CAD build for the part. Positions are in the model's coordinates, mm. A direction names the side the tool comes from. Give positions to 0.01 mm unless a question says otherwise; leave off trailing zeros. Loops run counter-clockwise (first coordinate to the right, second up) from the corner with the lowest first, then second, coordinate; pieces in that order, holes last. Notation, with made-up numbers: M -37,-15 L -8,-15 A18 cw -8,-6 Z; hole C 10,80 d9. An arc over 180 degrees is marked long. Answer as CSV lines item,"result".
from build123d import *

# Parameters (mm, degrees)
SKETCH1_W           = 12
SKETCH1_H           = 10
BOSS_EXTRUDE1_DEPTH = 40.48
SKETCH2_OUTSIDE_W   = 22.678
SKETCH2_OUTSIDE_H   = 20.678
CUT_EXTRUDE1_DEPTH  = 10
FILLET1_R           = 1


with BuildPart() as part:
    # Sketch1 → Boss-Extrude1 (new body)
    with BuildSketch(Plane.XY):
        Rectangle(SKETCH1_W, SKETCH1_H)
    extrude(amount=-BOSS_EXTRUDE1_DEPTH)

    # Sketch2 outside → Cut-Extrude1 (cut)
    with BuildSketch(Plane.XY):
        Rectangle(SKETCH2_OUTSIDE_W, SKETCH2_OUTSIDE_H)
        with BuildLine():
            Line((-1.118033989, 1), (1.118033989, 1))
            ThreePointArc((1.118033989, 1), (0, -1.5), (-1.118033989, 1))
        make_face(mode=Mode.SUBTRACT)
    extrude(amount=-CUT_EXTRUDE1_DEPTH, mode=Mode.SUBTRACT)

    # Fillet1
    fillet1_edges = [part.edges().sort_by_distance(p)[0] for p in [
        (-6, 5, -25.24),
        (6, 5, -25.24),
    ]]
    fillet(fillet1_edges, radius=FILLET1_R)


solid = part.part
1) Band-saw the part on D-D on y = 2.5. Give the cut face in (x, z).
Answer below:
outline,"M -6,-40.48 L 6,-40.48 L 6,-10 L -6,-10 Z"
2) Flat gauge pins, fed straight in: pin 1 (2.5 mm diameter, centred on x = 0, z = -3, fed in from +Y); pin 2 (2 mm diameter, centred on x = -4, y = 2, fed in from +Z). Where does each tip first touch, or does it go through?
Answer below:
pin 1,"stops at y = 1"
pin 2,"stops at z = -10"
3) Which spindle directions (+Z, -Z, +X, -X, +Y, -Y) get a long thin tool onto all of the face, cutting with end or side? Do faces 1 (the face through (6, -1, -25)), 2 (the face through (0, 1, -5)), 3 (the face through (0, -1.5, -4.9)). Say none if no direction does.
Answer below:
face 1,"+Z, -Z, +X, +Y, -Y"
face 2,"+Z, +X, -X, +Y"
face 3,"+Z"
4) Drill centre lines: line 1 (Z direction, x = -5.5, y = -1); line 2 (X direction, y = -1, z = -9). Where is each one in solid material? Low to high. Write a range as from..to.
Answer below:
line 1,"z = -40.48..-10"
line 2,"x = -1.12..1.12"
5) Band-saw the part on A-A on x = 0. Give the cut face in (y, z), and give its area (3 significant figures).
Answer below:
outline,"M -5,-40.48 L 5,-40.48 L 5,-10 L 1,-10 L 1,0 L -1.5,0 L -1.5,-10 L -5,-10 Z"
area,"330 mm^2"
6) Band-saw the part on C-C on z = -4. Give the cut face in (x, y), and give its area (3 significant figures).
Answer below:
outline,"M -1.12,1 A1.5 ccw long 1.12,1 Z"
area,"6.29 mm^2"
7) Band-saw the part on B-B on y = 0. Give the cut face in (x, z), and give its area (3 significant figures).
Answer below:
outline,"M -6,-40.48 L 6,-40.48 L 6,-10 L 1.5,-10 L 1.5,0 L -1.5,0 L -1.5,-10 L -6,-10 Z"
area,"396 mm^2"
